Source: CAD feature listing. Evaluate the final solid. Frame: model axes, mm. A direction names the side the tool comes from. Coordinates: 2 decimals unless noted, no trailing zeros. Write each loop counter-clockwise with the first axis right and the second up, starting at its lowest first coordinate (ties: lowest second). Pieces come first, ordered by that corner, then holes. Notation, with made-up numbers: (51.25, 73) -> (104.25, 73) arc R14 ccw to (104.25, 80) -> close; hole circle Ø9 at (-12, -27). An arc over 180 degrees is marked (long way). Write item = value, one per line.
from build123d import *

# Parameters (mm, degrees)
SKETCH1_W           = 65.35
SKETCH1_H           = 35.35
BOSS_EXTRUDE1_DEPTH = 3.175
SKETCH2_W           = 28.175
SKETCH2_H           = 7.5
CUT_EXTRUDE1_DEPTH  = 4.175
SKETCH3_W           = 10
SKETCH3_H           = 3.175
SKETCH3_W_2         = 3.175
SKETCH3_H_2         = 7.5
SKETCH3_H_3         = 5.9125
SKETCH3_H_4         = 5.35
SKETCH3_H_5         = 1.5875
CUT_EXTRUDE2_DEPTH  = 3.175
SKETCH7_W           = 3.175
SKETCH7_H           = 10
CUT_EXTRUDE3_DEPTH  = 4.175
BOSS_EXTRUDE2_DEPTH = 3.175


with BuildPart() as part:
    # Sketch1 → Boss-Extrude1 (new body)
    with BuildSketch(Plane(origin=(0, 0, 0), x_dir=(1, 0, 0), z_dir=(0, 1, 0))):
        with Locations((32.675, 17.675)):
            Rectangle(SKETCH1_W, SKETCH1_H)
    extrude(amount=BOSS_EXTRUDE1_DEPTH)

    # Sketch2 → Cut-Extrude1 (cut, through all)
    with BuildSketch(Plane.XZ):
        with Locations((51.2625, -31.6)):
            Rectangle(SKETCH2_W, SKETCH2_H)
    extrude(amount=-CUT_EXTRUDE1_DEPTH, mode=Mode.SUBTRACT)

    # Sketch3 → Cut-Extrude2 (cut)
    with BuildSketch(Plane.XZ):
        with Locations((52.675, -1.5875)):
            Rectangle(SKETCH3_W, SKETCH3_H)
        with Locations((63.7625, -3.75)):
            Rectangle(SKETCH3_W_2, SKETCH3_H_2)
        with Locations((63.7625, -18.75)):
            Rectangle(SKETCH3_W_2, SKETCH3_H_2)
        with Locations((52.675, -26.2625)):
            Rectangle(SKETCH3_W, SKETCH3_H)
        Polygon((37.175, -27.85), (37.675, -27.85), (37.675, -24.675), (27.675, -24.675), (27.675, -27.85), (34, -27.85), align=None)
        with Locations((35.5875, -30.80625)):
            Rectangle(SKETCH3_W_2, SKETCH3_H_3)
        Polygon((37.175, -35.35), (37.175, -33.7625), (34, -33.7625), (27.675, -33.7625), (27.675, -35.35), align=None)
        with Locations((12.675, -26.2625)):
            Rectangle(SKETCH3_W, SKETCH3_H)
        with Locations((1.5875, -32.675)):
            Rectangle(SKETCH3_W_2, SKETCH3_H_4)
        with Locations((1.5875, -18.75)):
            Rectangle(SKETCH3_W_2, SKETCH3_H_2)
        with Locations((1.5875, -3.75)):
            Rectangle(SKETCH3_W_2, SKETCH3_H_2)
        with Locations((12.675, -1.5875)):
            Rectangle(SKETCH3_W, SKETCH3_H)
        with Locations((32.675, -1.5875)):
            Rectangle(SKETCH3_W, SKETCH3_H)
        with Locations((12.675, -34.55625)):
            Rectangle(SKETCH3_W, SKETCH3_H_5)
    extrude(amount=-CUT_EXTRUDE2_DEPTH, mode=Mode.SUBTRACT)

    # Sketch7 → Cut-Extrude3 (cut, through all)
    with BuildSketch(Plane.XZ):
        with Locations((11.0875, -11.825)):
            Rectangle(SKETCH7_W, SKETCH7_H)
        with Locations((54.2625, -11.825)):
            Rectangle(SKETCH7_W, SKETCH7_H)
    extrude(amount=-CUT_EXTRUDE3_DEPTH, mode=Mode.SUBTRACT)

    # Sketch6 → Boss-Extrude2 (add)
    with BuildSketch(Plane(origin=(0, 3.175, 0), x_dir=(1, 0, 0), z_dir=(0, 1, 0))):
        Polygon((7.929, -0.254), (7.929, 2.921), (17.421, 2.921), (17.421, -0.254), (27.929, -0.254), (27.929, 2.921), (37.421, 2.921), (37.421, -0.254), (47.929, -0.254), (47.929, 2.921), (57.421, 2.921), (57.421, -0.254), (62.429, -0.254), (62.429, 7.246), (65.604, 7.246), (65.604, 15.254), (62.429, 15.254), (62.429, 22.246), (65.604, 22.246), (65.604, 28.104), (57.421, 28.104), (57.421, 24.929), (47.929, 24.929), (47.929, 28.104), (37.421, 28.104), (37.421, 24.929), (27.929, 24.929), (27.929, 27.596), (34.254, 27.596), (34.254, 34.0165), (27.929, 34.0165), (27.929, 35.604), (17.421, 35.604), (17.421, 34.0165), (7.929, 34.0165), (7.929, 35.604), (2.921, 35.604), (2.921, 30.254), (-0.254, 30.254), (-0.254, 22.246), (2.921, 22.246), (2.921, 15.254), (-0.254, 15.254), (-0.254, 7.246), (2.921, 7.246), (2.921, -0.254), align=None)
        Polygon((6.675, 4.175), (18.675, 4.175), (18.675, 1), (26.675, 1), (26.675, 4.175), (38.675, 4.175), (38.675, 1), (46.675, 1), (46.675, 4.175), (58.675, 4.175), (58.675, 1), (61.175, 1), (61.175, 8.5), (64.35, 8.5), (64.35, 14), (61.175, 14), (61.175, 23.5), (64.35, 23.5), (64.35, 26.85), (58.675, 26.85), (58.675, 23.675), (46.675, 23.675), (46.675, 26.85), (38.675, 26.85), (38.675, 23.675), (26.675, 23.675), (26.675, 28.85), (33, 28.85), (33, 32.7625), (26.675, 32.7625), (26.675, 34.35), (18.675, 34.35), (18.675, 32.7625), (6.675, 32.7625), (6.675, 34.35), (4.175, 34.35), (4.175, 29), (1, 29), (1, 23.5), (4.175, 23.5), (4.175, 14), (1, 14), (1, 8.5), (4.175, 8.5), (4.175, 1), (6.675, 1), align=None, mode=Mode.SUBTRACT)
    extrude(amount=-BOSS_EXTRUDE2_DEPTH)


solid = part.part
1) Material intervals for probe 1 along X at (y, z) = (0.5, -8) (3 decimals); probe 2 along X at (y, z) = (0.95, -25.5) (3 decimals); probe 3 along X at (y, z) = (2.7, -2), sorted ascending. Write a range as [from, to].
Answer block:
probe_1 = [-0.254, 9.5], [12.675, 52.675], [55.85, 65.604]
probe_2 = [-0.254, 7.675], [17.675, 27.929], [37.421, 47.929], [57.421, 65.604]
probe_3 = [2.92, 7.93], [17.42, 27.93], [37.42, 47.93], [57.42, 62.43]
2) Reachability of faces 4 (the flat face through (43, 2, -28.104)), 5 (the flat face through (7.675, 2, -26)), 6 (the flat face through (57.421, 2, -1)), 7 (the flat face through (2.921, 2, -33)), 8 (the flat face through (17.421, 2, -35)) from +Z, -Z, +X, -X, +Y, -Y: full face, straight path, thin tool, end or side. Return the list, or none.
Answer block:
face_4 = -Z, +X, +Y, -Y
face_5 = +Y, -Y
face_6 = +Z, +Y, -Y
face_7 = -Z, -X, +Y, -Y
face_8 = -Z, +Y, -Y
3) Cut plane A-A, the plane x = 54.5. Output: boundary loops of the cut face in (y, z) (3 decimals).
Answer block:
outline = (0, -24.929) -> (3.175, -24.929) -> (3.175, -16.825) -> (0, -16.825) -> close; (0, -6.825) -> (3.175, -6.825) -> (3.175, -2.921) -> (0, -2.921) -> close
4) Cut plane C-C, the plane x = 31. Output: boundary loops of the cut face in (y, z) (1 decimal).
Answer block:
outline = (0, -34) -> (3.2, -34) -> (3.2, -27.6) -> (0, -27.6) -> close; (0, -24.9) -> (3.2, -24.9) -> (3.2, -2.9) -> (0, -2.9) -> close
5) Cut plane B-B, the plane z = -2. Output: boundary loops of the cut face in (x, y) (3 decimals), and give its area (3 significant figures).
Answer block:
outline = (2.921, 0) -> (7.929, 0) -> (7.929, 3.175) -> (2.921, 3.175) -> close; (17.421, 0) -> (27.929, 0) -> (27.929, 3.175) -> (17.421, 3.175) -> close; (37.421, 0) -> (47.929, 0) -> (47.929, 3.175) -> (37.421, 3.175) -> close; (57.421, 0) -> (62.429, 0) -> (62.429, 3.175) -> (57.421, 3.175) -> close
area = 98.5 mm2
6) Cut plane D-D, the plane y = 0.8. Give the number of separate pieces and of enclosed holes in the cut face, and give its area (3 significant figures).
Answer block:
separate_pieces = 1
enclosed_holes = 3
area = 1,750 mm2
7) Pull-direction query (Z, two-part tool) for faces 1 (the flat face through (65.604, 2, -11)), 2 (the flat face through (62.429, 2, -19)), 3 (the flat face through (5, 2, -35.604)); classes: +Z half, -Z half, draft (parallel to the pull), parting line (faces both ways), or undercut.
Answer block:
face_1 = draft
face_2 = undercut
face_3 = -Z half
8) First-contact query: pin 1 Ø1 at (y, z) = (1, -1) entering from -X; pin 2 Ø1.6 at (x, y) = (32.5, 1.5) entering from -Z; pin 3 Ø1 at (x, y) = (31.5, 1) entering from +Z; pin 4 Ø8 at (x, z) = (54, -29.5) entering from +Y (3 decimals). Flat tips, straight axial feed; report the tip coordinate or a pass-through.
Answer block:
pin_1 = 2.92
pin_2 = -34.02
pin_3 = -2.92
pin_4 = 3.175
